Geometry check sheet. Reference: the model listing, model coordinates, mm. Face numbers are marked on the shaded views. A direction names the side the tool comes from. Coordinates: 2 decimals unless noted, no trailing zeros. Loops run counter-clockwise (first coordinate to the right, second up) from the corner with the lowest first, then second, coordinate; pieces in that order, holes last.
from build123d import *

# Parameters (mm, degrees)
SKETCH_1_W               = 18.5
SKETCH_1_H               = 18.5
EXTRUDE_2_DEPTH          = 10
CUT_EXTRUDE_1_DEPTH      = 8
CUT_EXTRUDE_1_DEPTH_BACK = 10
SKETCH_1_5_W             = 15
SKETCH_1_5_H             = 15
SKETCH_1_8_R             = 3
EXTRUDE_3_DEPTH          = 8


with BuildPart() as part:
    # 草图1 → 凸台-拉伸2 (new body)
    with BuildSketch(Plane(origin=(-54.452348576, 0, -10.111307481), x_dir=(1, 0, 0), z_dir=(0, 1, 0))):
        with Locations((-0.232982833, 0.198747616)):
            Rectangle(SKETCH_1_W, SKETCH_1_H)
    extrude(amount=EXTRUDE_2_DEPTH)

    # 草图1<5> → 切除-拉伸1 (cut, two sides: drawn at the far end of the back side and taken through both)
    with BuildSketch(Plane(origin=(-54.452348576, 0, -10.111307481), x_dir=(1, 0, 0), z_dir=(0, 1, 0)).offset(-CUT_EXTRUDE_1_DEPTH_BACK)):
        with Locations((-0.232977593, 0.198745421)):
            Rectangle(SKETCH_1_5_W, SKETCH_1_5_H)
    extrude(amount=CUT_EXTRUDE_1_DEPTH + CUT_EXTRUDE_1_DEPTH_BACK, mode=Mode.SUBTRACT)


with BuildPart() as body_2:
    # 草图1<8> → 凸台-拉伸3 (new body)
    with BuildSketch(Plane(origin=(-54.452348576, 0, -10.111307481), x_dir=(1, 0, 0), z_dir=(0, 1, 0))):
        with Locations(Location((-32.631590837, 12.584276694, 0), (0, 0, 270))):
            Circle(SKETCH_1_8_R)
        Polygon((-34.631589769, 12.124234893), (-34.631589769, 13.124234893), (-33.131574719, 13.124234893), (-33.131574719, 14.5842993), (-32.131574719, 14.5842993), (-32.131574719, 13.124234893), (-30.631589769, 13.124234893), (-30.631589769, 12.124234893), (-32.131574719, 12.124234893), (-32.131574719, 10.5842993), (-33.131574719, 10.5842993), (-33.131574719, 12.124234893), align=None, mode=Mode.SUBTRACT)
    extrude(amount=EXTRUDE_3_DEPTH)


solid = part.part
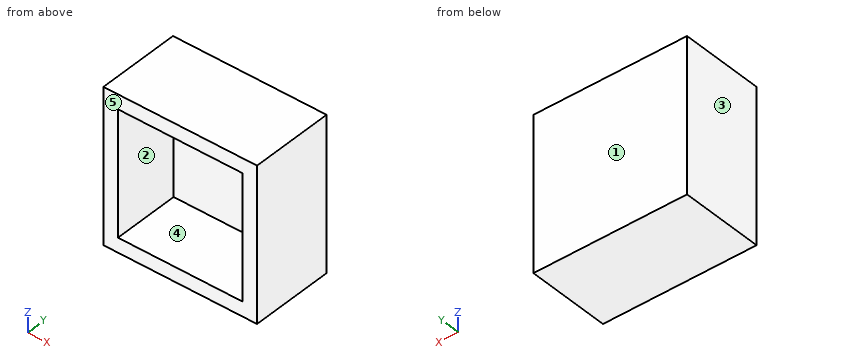
(1) Sectioned sample at C-C on z = -14. Record the cut outline in (x, y).
Findings:
outline: (-63.94, 0) - (-62.19, 0) - (-62.19, 8) - (-47.19, 8) - (-47.19, 0) - (-45.44, 0) - (-45.44, 10) - (-63.94, 10) - close
(2) Sectioned sample at A-A on y = 6.25. Record the cut outline in (x, z).
Findings:
outline: (-63.94, -19.56) - (-45.44, -19.56) - (-45.44, -1.06) - (-63.94, -1.06) - close; hole (-62.19, -17.81) - (-47.19, -17.81) - (-47.19, -2.81) - (-62.19, -2.81) - close
(3) Gauge pin test, flat end, axial feed: pin 1 Ø5 at (x, z) = (-53, -10.5) entering from -Y. Record the tip position at first contact, or that the pin passes through.
Findings:
pin 1: stops at y = 8
(4) Sectioned sample at B-B on x = -57. Record the cut outline in (y, z), and give its area (3 significant figures).
Findings:
outline: (0, -19.56) - (10, -19.56) - (10, -1.06) - (0, -1.06) - (0, -2.81) - (8, -2.81) - (8, -17.81) - (0, -17.81) - close
area: 65.0 mm2
(5) Scan lines: L1, parallel to X at y = 0.75, z = -15.5; L2, parallel to Z at x = -57.5, y = 1.75; L3, parallel to Y at x = -50.5, z = -12. Record each from-to range of solid material in increasing order.
Findings:
L1: x = -63.94 to -62.19, -47.19 to -45.44
L2: z = -19.56 to -17.81, -2.81 to -1.06
L3: y = 8 to 10
(6) Access from +Z, -Z, +X, -X, +Y, -Y to the whole of each face (thin tool, end or side, straight path). Record for the marked faces 4 and 5.
Findings:
face 4: -Y
face 5: +Z, -Z, +X, -X, -Y
(7) Draft check along X on the marked faces 1, 2 and 3. Enter one of: +X half, -X half, draft (parallel to the pull), parting line (faces both ways), or undercut.
Findings:
face 1: draft
face 2: undercut
face 3: -X half
